from build123d import *

# Parameters (mm, degrees)
SKETCH1_R           = 1.4224
BOSS_EXTRUDE1_DEPTH = 3.048


with BuildPart() as part:
    # Sketch1 → Boss-Extrude1 (new body)
    # profile 1 of 3: a face of its own
    with BuildSketch(Plane(origin=(0, 0, 0), x_dir=(1, 0, 0), z_dir=(0, 1, 0))):
        with BuildLine():
            Line((5.703787569, 57.336566523), (-2.983524071, 33.468373955))
            ThreePointArc((-2.983524071, 33.468373955), (0.551332964, 35.509224616), (3.175, 32.38246))
            Line((3.175, 32.38246), (3.175, 31.822621836))
            Line((3.175, 31.822621836), (11.670835711, 55.164738613))
            ThreePointArc((11.670835711, 55.164738613), (9.773225596, 59.234176639), (5.703787569, 57.336566523))
        make_face()
        with Locations(Location((8.68731164, 56.250652568, 0), (0, 0, 90))):
            Circle(SKETCH1_R, mode=Mode.SUBTRACT)
    # profile 2 of 3: a face of its own
    with BuildSketch(Plane(origin=(0, 0, 0), x_dir=(1, 0, 0), z_dir=(0, 1, 0))):
        with BuildLine():
            ThreePointArc((-2.983524071, 33.468373955), (-3.126764616, 32.933792964), (-3.175, 32.38246))
            ThreePointArc((-3.175, 32.38246), (-0.551332964, 29.255695384), (2.983524071, 31.296546045))
            Line((2.983524071, 31.296546045), (3.175, 31.822621836))
            Line((3.175, 31.822621836), (3.175, 32.38246))
            ThreePointArc((3.175, 32.38246), (0.551332964, 35.509224616), (-2.983524071, 33.468373955))
        make_face()
        with Locations(Location((0, 32.38246, 0), (0, 0, 90))):
            Circle(SKETCH1_R, mode=Mode.SUBTRACT)
    # profile 3 of 3: a face of its own
    with BuildSketch(Plane(origin=(0, 0, 0), x_dir=(1, 0, 0), z_dir=(0, 1, 0))):
        with BuildLine():
            Line((-3.175, 32.38246), (-3.175, 0))
            ThreePointArc((-3.175, 0), (0, -3.175), (3.175, 0))
            Line((3.175, 0), (3.175, 31.822621836))
            Line((3.175, 31.822621836), (2.983524071, 31.296546045))
            ThreePointArc((2.983524071, 31.296546045), (-0.551332964, 29.255695384), (-3.175, 32.38246))
        make_face()
        with Locations(Location((0, 0, 0), (0, 0, 90))):
            Circle(SKETCH1_R, mode=Mode.SUBTRACT)
    extrude(amount=BOSS_EXTRUDE1_DEPTH)


solid = part.part
Can you work these out from the model? Positions are in its coordinate system, mm. A direction names the side the tool comes from. Give positions to 0.01 mm unless a question says otherwise; leave off trailing zeros. Order: outer loops, then holes, each group sorted by start corner. A loop starts at its lowest first (then second) coordinate and runs counter-clockwise, first axis right, second up. Notation, with made-up numbers: M 46.25,24 L 84.25,24 A25 ccw 84.25,50 Z; hole C 70,-12.5 d2. An arc over 180 degrees is marked long. Use a Markdown table: item, result. Add a question column.
Item 1: Will these pins go through, and if not, where does the flat tip stop? pin 1 (4.5 mm diameter, centred on x = 8.69, z = -56.25, fed in from +Y); pin 2 (1.5 mm diameter, centred on y = 1, z = -28, fed in from +X) (3 decimals); pin 3 (2.5 mm diameter, centred on x = 0, z = 0, fed in from -Y).
Item 2: Suppose I cut it at C-C (z = -23). List the corners of the cut face in (x, y) for me (3 decimals), then the cut area to 3 significant figures.
Item 3: We'd pull the mould along X, two halves only. Please class faces 3 (the flat face through (1.42, 1.5, -45.57)), 4 (the cylindrical face through (9.232, 1.503, -57.565)), 5 (the flat face through (3, 3.048, -29)), 6 (the cylindrical face through (-0.06, 1.5, -30.96)): +X half, -X half, draft (parallel to the pull), parting line (faces both ways), or undercut.
Item 4: For faces 1 (the flat face through (3.175, 2, -16)), 2 (the cylindrical face through (1.39, 1.5, 0.31)), which set-ups out of +Z, -Z, +X, -X, +Y, -Y let a thin tool reach every point of the face, with its end or its side?
Item 5: Suppose I cut it at D-D (z = -39). List the corners of the cut face in (x, y) for me, then the cut area to 3 significant figures.
Item 6: If I drill on L1, parallel to X at y = 0.6, z = -7 (3 decimals); L2, parallel to X at y = 1.9, z = -56.5; L3, parallel to X at y = 1.25, z = -37.5, over which ranges is the centre line in solid material (lowest first)? Write a range as [from, to].
Item 7: Suppose I cut it at B-B (y = 0.95). List the corners of the cut face in (x, z) for me (3 decimals), then the cut area to 3 significant figures.
Item 8: Suppose I cut it at A-A (x = 0). List the corners of the cut face in (y, z) for me (3 decimals).
Answer sheet:
| question | item | result |
|---|---|---|
| 1 | pin 1 | stops at y = 3.05 |
| 1 | pin 2 | stops at x = 3.175 |
| 1 | pin 3 | passes through |
| 2 | outline | M -3.175,0 L 3.175,0 L 3.175,3.048 L -3.175,3.048 Z |
| 2 | area | 19.4 mm² |
| 3 | face 3 | -X half |
| 3 | face 4 | undercut |
| 3 | face 5 | draft |
| 3 | face 6 | undercut |
| 4 | face 1 | +Z, +X, +Y, -Y |
| 4 | face 2 | +Y, -Y |
| 5 | outline | M -0.97,0 L 5.79,0 L 5.79,3.05 L -0.97,3.05 Z |
| 5 | area | 20.6 mm² |
| 6 | L1 | x = [-3.175, 3.175] |
| 6 | L2 | x = [5.4, 7.29], [10.09, 11.85] |
| 6 | L3 | x = [-1.52, 5.24] |
| 7 | outline | M -3.175,-32.382 A3.175 ccw -2.984,-33.468 L 5.704,-57.337 A3.175 ccw 11.671,-55.165 L 3.175,-31.823 L 3.175,0 A3.175 ccw -3.175,0 Z; hole C 0,-32.382 d2.845; hole C 0,0 d2.845; hole C 8.687,-56.251 d2.845 |
| 7 | area | 380 mm² |
| 8 | outline | M 0,-41.666 L 3.048,-41.666 L 3.048,-33.805 L 0,-33.805 Z; M 0,-30.96 L 3.048,-30.96 L 3.048,-1.422 L 0,-1.422 Z; M 0,1.422 L 3.048,1.422 L 3.048,3.175 L 0,3.175 Z |
